Answer from the drawing. Dimensions are ordinates in mm from the lowest x, y and z of the part. A direction names the side the tool comes from. Give positions to 0.01 mm unless a question says otherwise; leave off trailing zeros. Order: outer loops, then holes, each group sorted by start corner. A loop starts at its lowest first (then second) coordinate and runs counter-clockwise, first axis right, second up. Notation, with made-up numbers: (39, -22) - (53, -22) arc R19 ccw to (53, -5) - close; hole circle Ø6 at (44.5, 8). An arc over 180 degrees is marked (long way). Use a Markdown table: item, result. Add a question column.
1) The mould has two halves that part along Z. Classify the marked faces 1, 2, 3 and 4: released by +Z, released by -Z, zero draft, split by the parting line, or undercut.
2) Find section C-C, the plane y = 8. Determine the outline of the cut face in (x, z), plus the area to 3 significant figures.
3) For the marked faces 5, 6 and 7, determine the directions among +Z, -Z, +X, -X, +Y, -Y from which every point of the face is accessible in a straight line to the end or side of a thin tool.
4) Find section D-D, the plane z = 14. Determine the outline of the cut face in (x, y).
5) Find section B-B, the plane z = 21.5. Determine the outline of the cut face in (x, y), plus the area to 3 significant figures.
6) Flat-ended cylindrical pins translate along their axes: pin 1 (1.8 mm diameter, centred on x = 60, y = 8, fed in from +Z); pin 2 (8 mm diameter, centred on y = 45, z = 26, fed in from -X); pin 3 (2 mm diameter, centred on x = 26, z = 25, fed in from -Y); pin 4 (6 mm diameter, centred on x = 64, y = 8.5, fed in from +Z). Find the tip coordinate at first contact, or state that the pin passes through.
7) Straight lines are drawn through the part: line 1 (X direction, y = 53.65, z = 21.5); line 2 (X direction, y = 37.5, z = 28.5); line 3 (Z direction, x = 72.5, y = 51). For each, find the intervals that lie inside material, in ascending order.
8) Find section A-A, the plane x = 27.5. Determine the outline of the cut face in (y, z).
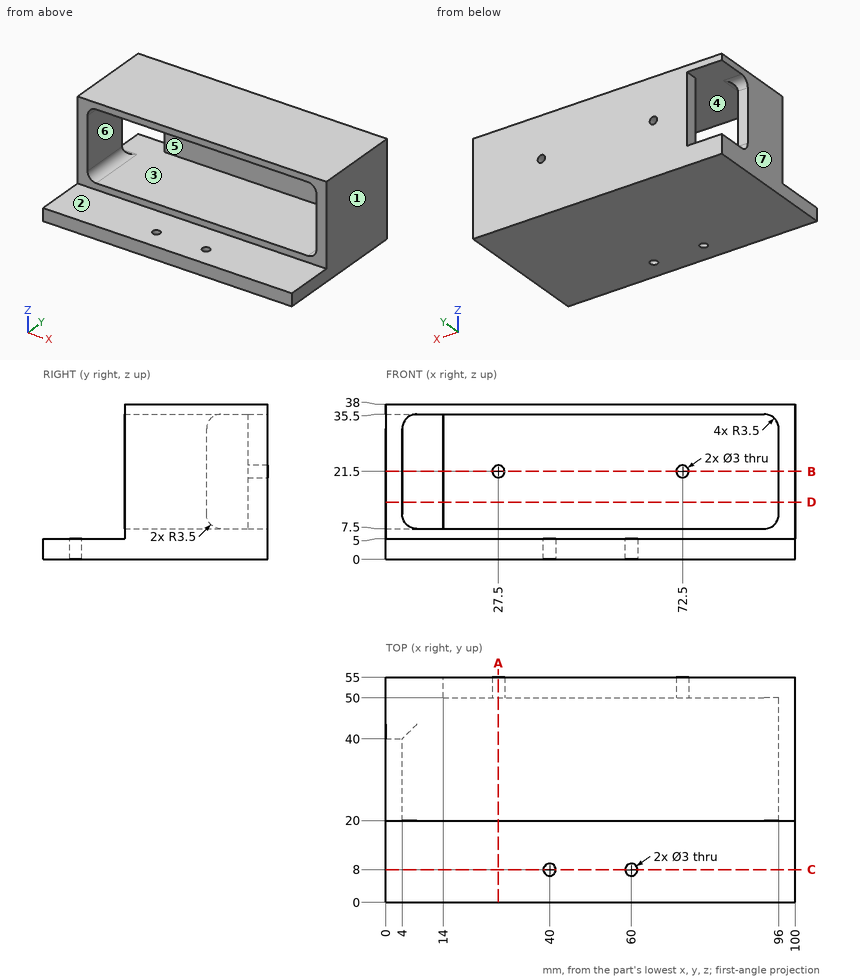
The answers:
| question | item | result |
|---|---|---|
| 1 | face 1 | zero draft |
| 1 | face 2 | released by +Z |
| 1 | face 3 | undercut |
| 1 | face 4 | undercut |
| 2 | outline | (0, 0) - (38.5, 0) - (38.5, 5) - (0, 5) - close; (41.5, 0) - (58.5, 0) - (58.5, 5) - (41.5, 5) - close; (61.5, 0) - (100, 0) - (100, 5) - (61.5, 5) - close |
| 2 | area | 470 mm2 |
| 3 | face 5 | -X, -Y |
| 3 | face 6 | +Y, -Y |
| 3 | face 7 | +Z, -Z, -X, +Y, -Y |
| 4 | outline | (0, 20) - (4, 20) - (4, 40) - (0, 40) - close; (14, 50) - (96, 50) - (96, 20) - (100, 20) - (100, 55) - (14, 55) - close |
| 5 | outline | (0, 20) - (4, 20) - (4, 40) - (0, 40) - close; (14, 50) - (26, 50) - (26, 55) - (14, 55) - close; (29, 50) - (71, 50) - (71, 55) - (29, 55) - close; (74, 50) - (96, 50) - (96, 20) - (100, 20) - (100, 55) - (74, 55) - close |
| 5 | area | 600 mm2 |
| 6 | pin 1 | through |
| 6 | pin 2 | x = 96 |
| 6 | pin 3 | y = 50 |
| 6 | pin 4 | z = 5 |
| 7 | line 1 | 14 to 26, 29 to 71, 74 to 100 |
| 7 | line 2 | 0 to 4, 96 to 100 |
| 7 | line 3 | 0 to 20, 23 to 38 |
| 8 | outline | (0, 0) - (55, 0) - (55, 20) - (50, 20) - (50, 7.5) - (20, 7.5) - (20, 5) - (0, 5) - close; (20, 35.5) - (50, 35.5) - (50, 23) - (55, 23) - (55, 38) - (20, 38) - close |
